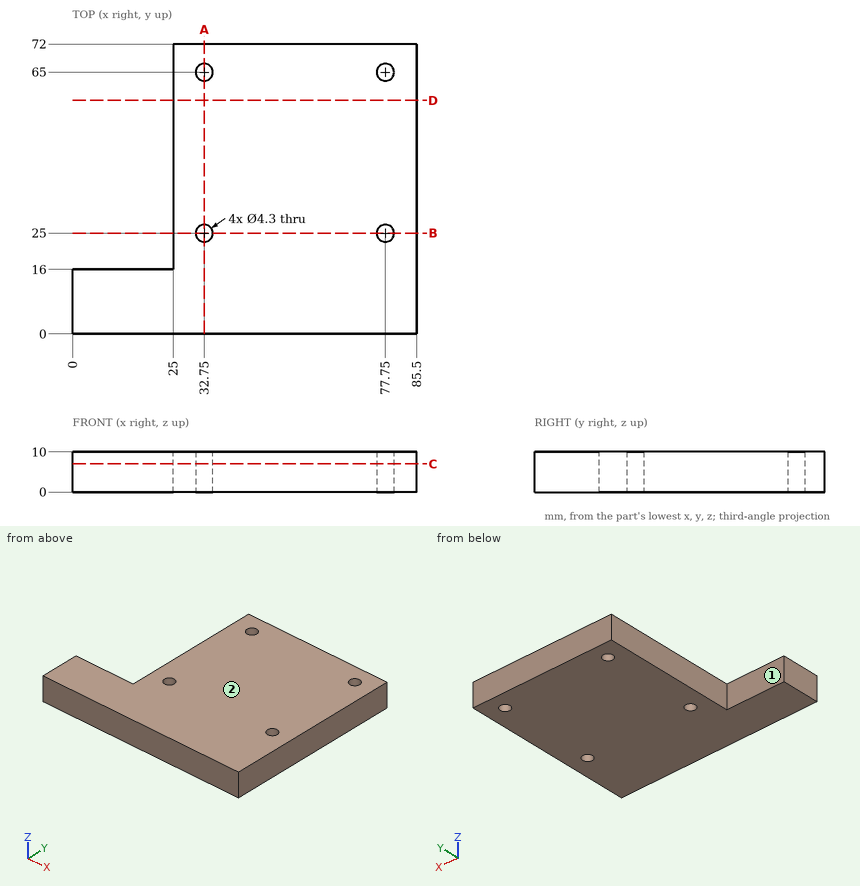
Input: dimensioned drawing with shaded views. Units: mm. Origin: part minimum x, y, z. A direction names the side the tool comes from. Coordinates: 2 decimals unless noted, no trailing zeros. Loops run counter-clockwise (first coordinate to the right, second up) from the corner with the lowest first, then second, coordinate; pieces in that order, holes last. Notation, with made-up numbers: M -26,72 L -18,72 A20 ccw -18,92 Z; hole C 1,-28.5 d10. An arc over 180 degrees is marked long. Use a Markdown table: item, result. Add a question column.
Q1. Section query D-D, the plane y = 58. Return loops of the section in (x, z).
Q2. Material intervals for L1, parallel to Y at x = 77.75, z = 6; L2, parallel to X at y = 16.5, z = 1.5, sorted ascending.
Q3. Access query for the marked faces 1 and 2. Directions: +Z, -Z, +X, -X, +Y, -Y. A direction counts if a zero-diameter tool reaches every point of the face in a straight line with its end or side. Return the directions, or none.
Q4. First-contact query: pin 1 (3 mm diameter, centred on y = 19, z = 9, fed in from -X); pin 2 (3.5 mm diameter, centred on x = 32.75, y = 25, fed in from -Z); pin 3 (3 mm diameter, centred on x = 12, z = 5, fed in from +Y). Flat tips, straight axial feed; report the tip coordinate or a pass-through.
Q5. Section query C-C, the plane z = 7. Return loops of the section in (x, y).
Q6. Section query B-B, the plane y = 25. Return loops of the section in (x, z), and give its area (3 significant figures).
Q7. Section query A-A, the plane x = 32.75. Return loops of the section in (y, z), and give its area (3 significant figures).
Result:
| question | item | result |
|---|---|---|
| 1 | outline | M 25,0 L 85.5,0 L 85.5,10 L 25,10 Z |
| 2 | L1 | y = 0 to 22.85, 27.15 to 62.85, 67.15 to 72 |
| 2 | L2 | x = 25 to 85.5 |
| 3 | face 1 | +Z, -Z, -X, +Y |
| 3 | face 2 | +Z, +X, -X, +Y, -Y |
| 4 | pin 1 | stops at x = 25 |
| 4 | pin 2 | passes through |
| 4 | pin 3 | stops at y = 16 |
| 5 | outline | M 0,0 L 85.5,0 L 85.5,72 L 25,72 L 25,16 L 0,16 Z; hole C 32.75,25 d4.3; hole C 32.75,65 d4.3; hole C 77.75,25 d4.3; hole C 77.75,65 d4.3 |
| 6 | outline | M 25,0 L 30.6,0 L 30.6,10 L 25,10 Z; M 34.9,0 L 75.6,0 L 75.6,10 L 34.9,10 Z; M 79.9,0 L 85.5,0 L 85.5,10 L 79.9,10 Z |
| 6 | area | 519 mm2 |
| 7 | outline | M 0,0 L 22.85,0 L 22.85,10 L 0,10 Z; M 27.15,0 L 62.85,0 L 62.85,10 L 27.15,10 Z; M 67.15,0 L 72,0 L 72,10 L 67.15,10 Z |
| 7 | area | 634 mm2 |
